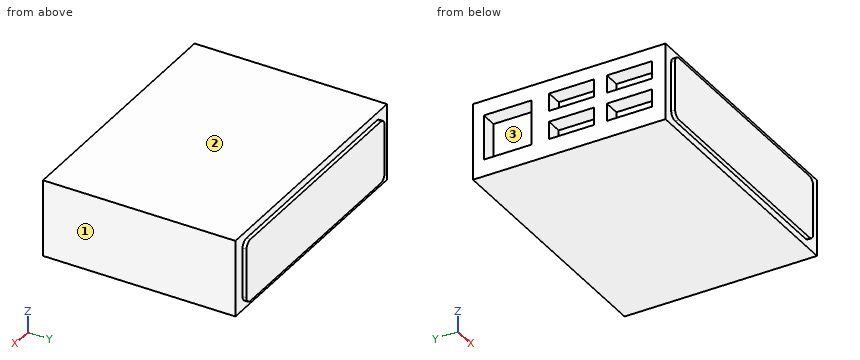
from build123d import *

# Parameters (mm, degrees)
F0_W     = 100
F0_H     = 75
F1_DEPTH = 30
F3_DEPTH = 1.524
F5_DEPTH = 1.524
F6_W     = 18.507942
F6_H     = 17.525221
F6_W_2   = 17.525221
F6_H_2   = 6.879058
F6_W_3   = 17.525222
F6_H_3   = 6.879059
F7_DEPTH = 6.35


with BuildPart() as f1:
    # F0 (on Top) → F1 (new body)
    with BuildSketch(Plane.XY):
        Rectangle(F0_W, F0_H)
    extrude(amount=F1_DEPTH)

    # F2 (on face) → F3 (join)
    with BuildSketch(Plane.XZ.offset(37.5)):
        with BuildLine():
            Line((42.337663, 27.106768), (-43.647963, 27.106768))
            ThreePointArc((-43.647963, 27.106768), (-45.444015, 26.362819), (-46.187963, 24.566768))
            Line((-46.187963, 24.566768), (-46.187963, 5.242487))
            ThreePointArc((-46.187963, 5.242487), (-45.444015, 3.446436), (-43.647963, 2.702487))
            Line((-43.647963, 2.702487), (42.337663, 2.702487))
            ThreePointArc((42.337663, 2.702487), (44.133714, 3.446436), (44.877663, 5.242487))
            Line((44.877663, 5.242487), (44.877663, 24.566768))
            ThreePointArc((44.877663, 24.566768), (44.133714, 26.362819), (42.337663, 27.106768))
        make_face()
    extrude(amount=F3_DEPTH)

    # F4 (on face) → F5 (join)
    with BuildSketch(Plane(origin=(0, 37.5, 0), x_dir=(-1, 0, 0), z_dir=(0, 1, 0))):
        with BuildLine():
            Line((43.245368, 27.151501), (-42.740258, 27.151501))
            ThreePointArc((-42.740258, 27.151501), (-44.53631, 26.407552), (-45.280258, 24.611501))
            Line((-45.280258, 24.611501), (-45.280258, 5.287221))
            ThreePointArc((-45.280258, 5.287221), (-44.53631, 3.491169), (-42.740258, 2.747221))
            Line((-42.740258, 2.747221), (43.245368, 2.747221))
            ThreePointArc((43.245368, 2.747221), (45.041419, 3.491169), (45.785368, 5.287221))
            Line((45.785368, 5.287221), (45.785368, 24.611501))
            ThreePointArc((45.785368, 24.611501), (45.041419, 26.407552), (43.245368, 27.151501))
        make_face()
    extrude(amount=F5_DEPTH)

    # F6 (on face) → F7 (cut)
    with BuildSketch(Plane(origin=(-50, 0, 0), x_dir=(0, -1, 0), z_dir=(-1, 0, 0))):
        with Locations((-23.994811, 15.395988)):
            Rectangle(F6_W, F6_H)
        with Locations((0.900829, 10.072907)):
            Rectangle(F6_W_2, F6_H_2)
        with Locations((0.947953, 21.248168)):
            Rectangle(F6_W_3, F6_H_3)
        with Locations((23.416942, 10.046705)):
            Rectangle(F6_W_2, F6_H_3)
        with Locations((23.464066, 21.221965)):
            Rectangle(F6_W_3, F6_H_3)
    extrude(amount=-F7_DEPTH, mode=Mode.SUBTRACT)


solid = f1.part
Source: CAD feature listing. Evaluate the final solid. Frame: model axes, mm. Face numbers are marked on the shaded views. Coordinates: 2 decimals unless noted, no trailing zeros. Loops run counter-clockwise (first coordinate to the right, second up) from the corner with the lowest first, then second, coordinate; pieces in that order, holes last. Notation, with made-up numbers: (41.5, -36.75) - (85.5, -36.75) arc R19 ccw to (85.5, -21.75) - close; hole circle Ø9 at (-12, -27). An arc over 180 degrees is marked (long way). One line per item, written item: value. Start each with the question number.
1. Ray query, L1, parallel to X at y = -2.5, z = 11; L2, parallel to Y at x = 46, z = 13.5. Return the intervals inside material, ascending.
2. Section B-B (y = 17). Return the cut outline in (x, z), and give its area (3 significant figures).
3. Mould query, pull axis Z, two halves, no side actions, for the marked faces 1, 2 and 3. Classes: pulls with the +Z half, pulls with the -Z half, needs draft (parallel to the pull), parting line crosses it, or undercut.
4. Section D-D (z = 28.25). Return the cut outline in (x, y).
5. Section A-A (z = 21). Return the cut outline in (x, y), and give its area (3 significant figures).
6. Contact query for flat-ended pins moving along their axis: P1, Ø7, axis at x = -47, z = 14.5, coming from the -Y side; P2, Ø0.5, axis at y = -38.5, z = 10, coming from the -X side; P3, Ø0.8, axis at x = 17, y = -38, coming from the +Z side; P4, Ø1.2, axis at y = 38.5, z = 13, coming from the -X side. Output: stop coordinate, or through.
7. Section C-C (y = -25). Return the cut outline in (x, z), and give its area (3 significant figures).
Verdict:
1. L1: x = -43.65 to 50
1. L2: y = -37.5 to 37.5
2. outline: (-50, 0) - (50, 0) - (50, 30) - (-50, 30) - (-50, 24.16) - (-43.65, 24.16) - (-43.65, 6.63) - (-50, 6.63) - close
2. area: 2,890 mm2
3. face 1: needs draft
3. face 2: pulls with the +Z half
3. face 3: undercut
4. outline: (-50, -37.5) - (50, -37.5) - (50, 37.5) - (-50, 37.5) - close
5. outline: (-50, -37.5) - (-46.19, -37.5) - (-46.19, -39.02) - (44.88, -39.02) - (44.88, -37.5) - (50, -37.5) - (50, 37.5) - (45.28, 37.5) - (45.28, 39.02) - (-45.79, 39.02) - (-45.79, 37.5) - (-50, 37.5) - (-50, 33.25) - (-43.65, 33.25) - (-43.65, 14.74) - (-50, 14.74) - (-50, 7.81) - (-43.65, 7.81) - (-43.65, -9.71) - (-50, -9.71) - (-50, -14.7) - (-43.65, -14.7) - (-43.65, -32.23) - (-50, -32.23) - close
5. area: 7,440 mm2
6. P1: stops at y = -39.02
6. P2: stops at x = -46.19
6. P3: stops at z = 27.11
6. P4: stops at x = -45.79
7. outline: (-50, 0) - (50, 0) - (50, 30) - (-50, 30) - (-50, 24.66) - (-43.65, 24.66) - (-43.65, 17.78) - (-50, 17.78) - (-50, 13.49) - (-43.65, 13.49) - (-43.65, 6.61) - (-50, 6.61) - close
7. area: 2,910 mm2
